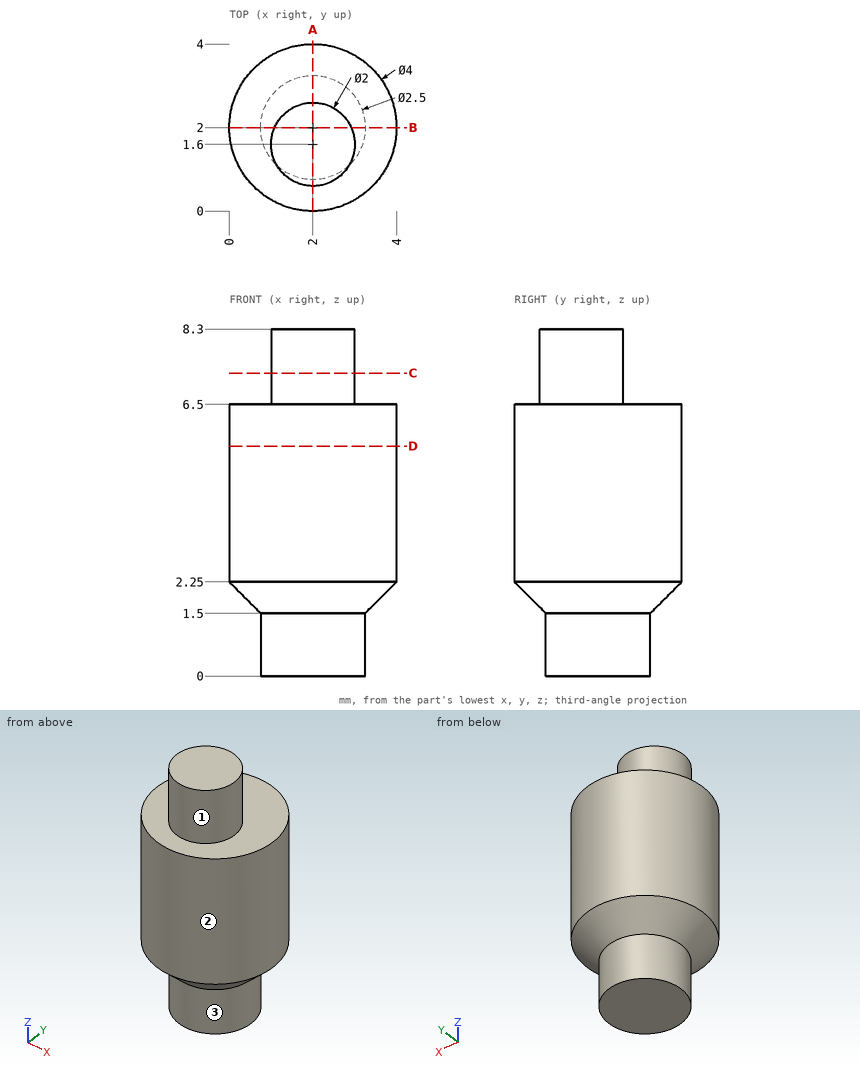
Design review of the part shown in the three views and the two pictorial views. Dimensions are in mm from the part's minimum x, y and z. A direction names the side the tool comes from. Round coordinates to 2 decimals unless told otherwise and drop trailing zeros. Write each loop counter-clockwise with the first axis right and the second up, starting at its lowest first coordinate (ties: lowest second). Pieces come first, ordered by that corner, then holes.
1) For line 1 along X through (y, z) = (1.3, 2.5); line 2 along Z through (x, y) = (0.8, 3.25); line 3 along Z through (x, y) = (3.55, 1.55), list the stretches that pass through material, from the lowest coordinate up.
Answer below:
line 1: x = 0.13 to 3.87
line 2: z = 1.98 to 6.5
line 3: z = 1.86 to 6.5
2) Machinability: for the marked faces 1, 2 and 3, which of the approach directions +Z, -Z, +X, -X, +Y, -Y give a long, thin tool a straight path to every point of the face, cutting with its end or side? Answer none if there is none.
Answer below:
face 1: +Z
face 2: +Z, -Z
face 3: -Z
3) Take a section at D-D on z = 5.5. Give the boundary of the cut face in (x, y).
Answer below:
outline: circle Ø4 at (2, 2)
4) Take a section at A-A on x = 2. Give the boundary of the cut face in (y, z).
Answer below:
outline: (0, 2.25) - (0.75, 1.5) - (0.75, 0) - (3.25, 0) - (3.25, 1.5) - (4, 2.25) - (4, 6.5) - (2.6, 6.5) - (2.6, 8.3) - (0.6, 8.3) - (0.6, 6.5) - (0, 6.5) - close
5) Take a section at B-B on y = 2. Give the boundary of the cut face in (x, z), then the cut area to 3 significant figures.
Answer below:
outline: (0, 2.25) - (0.75, 1.5) - (0.75, 0) - (3.25, 0) - (3.25, 1.5) - (4, 2.25) - (4, 6.5) - (2.92, 6.5) - (2.92, 8.3) - (1.08, 8.3) - (1.08, 6.5) - (0, 6.5) - close
area: 26.5 mm2
6) Take a section at C-C on z = 7.25. Give the boundary of the cut face in (x, y), then the cut area to 3 significant figures.
Answer below:
outline: circle Ø2 at (2, 1.6)
area: 3.14 mm2
7) Insertion check: pin 1 Ø1.5 at (x, z) = (1, 5.5) entering from +Y. The pin has a flat end and moves straight along its axis. Give the tip position at first contact, or say it passes through.
Answer below:
pin 1: stops at y = 3.98
